Can you work these out from the model? Positions are in its coordinate system, mm. Face numbers are marked on the shaded views. Give positions to 0.01 mm unless a question says otherwise; leave off trailing zeros. Order: outer loops, then holes, each group sorted by start corner. A loop starts at its lowest first (then second) coordinate and runs counter-clockwise, first axis right, second up. Notation, with made-up numbers: (10.5, 0) - (47.5, 0) arc R11 cw to (47.5, 16) - close; hole circle Ø6 at (81.5, -1). An arc over 180 degrees is marked (long way). Answer as a JSON object with one key per item and string values.
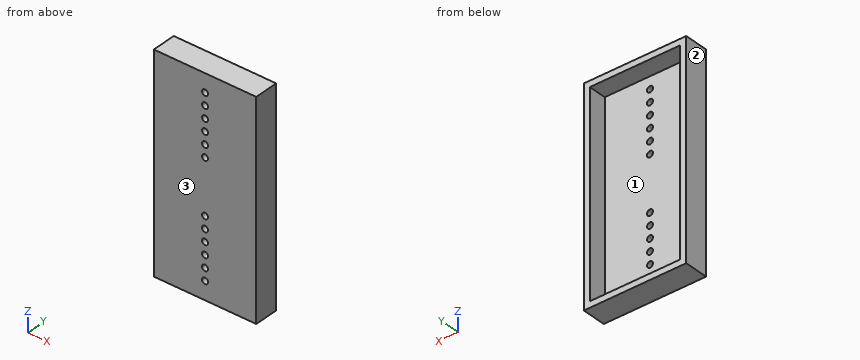
```python
from build123d import *

# Parameters (mm, degrees)
SKETCH_1_W          = 17
SKETCH_1_H          = 35
SKETCH_1_W_2        = 15
SKETCH_1_H_2        = 33
EXTRUDE_1_DEPTH     = 4
SKETCH_1_2_W        = 15
SKETCH_1_2_H        = 33
EXTRUDE_2_DEPTH     = 1
SKETCH_2_R          = 0.5
CUT_EXTRUDE_1_DEPTH = 20.862024066


with BuildPart() as part:
    # Sketch 1 → Extrude 1 (new body)
    with BuildSketch(Plane(origin=(0, 0, 0), x_dir=(1, 0, 0), z_dir=(0, 1, 0))):
        Rectangle(SKETCH_1_W, SKETCH_1_H)
        Rectangle(SKETCH_1_W_2, SKETCH_1_H_2, mode=Mode.SUBTRACT)
    extrude(amount=EXTRUDE_1_DEPTH)

    # Sketch 1_2 → Extrude 2 (add)
    with BuildSketch(Plane(origin=(0, 0, 0), x_dir=(1, 0, 0), z_dir=(0, 1, 0))):
        Rectangle(SKETCH_1_2_W, SKETCH_1_2_H)
    extrude(amount=EXTRUDE_2_DEPTH)

    # Sketch 2 → Cut-Extrude 1 (cut, through all)
    with BuildSketch(Plane.XZ):
        with Locations(Location((0, 14.5, 0), (0, 0, 270))):
            Circle(SKETCH_2_R)
        with Locations(Location((0, 12.5, 0), (0, 0, 270))):
            Circle(SKETCH_2_R)
        with Locations(Location((0, 10.5, 0), (0, 0, 270))):
            Circle(SKETCH_2_R)
        with Locations(Location((0, 8.5, 0), (0, 0, 270))):
            Circle(SKETCH_2_R)
        with Locations(Location((0, 6.5, 0), (0, 0, 270))):
            Circle(SKETCH_2_R)
        with Locations(Location((0, 4.5, 0), (0, 0, 270))):
            Circle(SKETCH_2_R)
        with Locations(Location((0, -4.5, 0), (0, 0, 90))):
            Circle(SKETCH_2_R)
        with Locations(Location((0, -6.5, 0), (0, 0, 90))):
            Circle(SKETCH_2_R)
        with Locations(Location((0, -8.5, 0), (0, 0, 90))):
            Circle(SKETCH_2_R)
        with Locations(Location((0, -10.5, 0), (0, 0, 90))):
            Circle(SKETCH_2_R)
        with Locations(Location((0, -12.5, 0), (0, 0, 90))):
            Circle(SKETCH_2_R)
        with Locations(Location((0, -14.5, 0), (0, 0, 90))):
            Circle(SKETCH_2_R)
    extrude(amount=-CUT_EXTRUDE_1_DEPTH, mode=Mode.SUBTRACT)


solid = part.part
```
Q1. If we section it at D-D, the plane z = 2.5: Please give me the cut outline in (x, y).
Recorded:
{"outline": "(-8.5, 0) - (8.5, 0) - (8.5, 4) - (7.5, 4) - (7.5, 1) - (-7.5, 1) - (-7.5, 4) - (-8.5, 4) - close"}
Q2. We'd pull the mould along X, two halves only. Please class the marked faces 1, 2 and 3: released by +X, released by -X, zero draft, split by the parting line, or undercut.
Recorded:
{"face 1": "undercut", "face 2": "released by -X", "face 3": "zero draft"}
Q3. I need wall thicknesses on L1, parallel to X at y = 2.5, z = -1; L2, parallel to Z at x = 6, y = 1.15; L3, parallel to X at y = 0.35, z = 4.5. Which ranges of each line are inside material? Lowest first, please.
Recorded:
{"L1": "x = -8.5 to -7.5, 7.5 to 8.5", "L2": "z = -17.5 to -16.5, 16.5 to 17.5", "L3": "x = -8.5 to -0.5, 0.5 to 8.5"}
Q4. If we section it at C-C, the plane y = 0.35: Count the separate pieces of the cut face and the enclosed holes in it, then the cut area to 3 significant figures.
Recorded:
{"separate pieces": "1", "enclosed holes": "12", "area": "586 mm^2"}
Q5. If we section it at A-A, the plane z = -14.5: Please give me the cut outline in (x, y).
Recorded:
{"outline": "(-8.5, 0) - (-0.5, 0) - (-0.5, 1) - (-7.5, 1) - (-7.5, 4) - (-8.5, 4) - close; (0.5, 0) - (8.5, 0) - (8.5, 4) - (7.5, 4) - (7.5, 1) - (0.5, 1) - close"}
Q6. If we section it at B-B, the plane x = -4.75: Please give me the cut outline in (y, z), then the cut area to 3 significant figures.
Recorded:
{"outline": "(0, -17.5) - (4, -17.5) - (4, -16.5) - (1, -16.5) - (1, 16.5) - (4, 16.5) - (4, 17.5) - (0, 17.5) - close", "area": "41.0 mm^2"}
Q7. I'm going to push a flat-ended pin straight in: pin 1 Ø1 at (x, z) = (6, -5.5) entering from +Y. Where does the tip first touch, or does it pass through?
Recorded:
{"pin 1": "stops at y = 1"}
